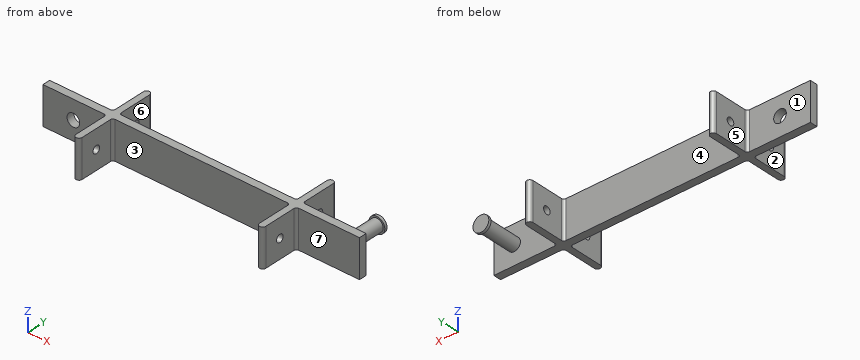
from build123d import *

# Parameters (mm, degrees)
BOSS_EXTRUDE1_DEPTH  = 30
FILLET1_R            = 2
FILLET2_RADIUS       = 2.5
FILLET2_LENGTH       = 30
FILLET3_RADIUS       = 2.5
FILLET3_LENGTH       = 30
FILLET4_R            = 2
SKETCH2_R            = 3
CUT_EXTRUDE4_DEPTH   = 163
SKETCH9_W            = 10
SKETCH9_H            = 6
BOSS_EXTRUDE8_DEPTH  = 30
SKETCH14_W           = 20
SKETCH14_H           = 6
BOSS_EXTRUDE12_DEPTH = 30
FILLET10_RADIUS      = 2.5
FILLET10_LENGTH      = 30
FILLET11_RADIUS      = 2.5
FILLET11_LENGTH      = 30
FILLET12_R           = 2
SKETCH16_R           = 3
CUT_EXTRUDE6_DEPTH   = 200
SKETCH17_W           = 30
SKETCH17_H           = 6
BOSS_EXTRUDE15_DEPTH = 30
SKETCH20_R           = 5
BOSS_EXTRUDE16_DEPTH = 36
SKETCH21_R           = 6.25
BOSS_EXTRUDE17_DEPTH = 2
SKETCH22_R           = 5
CUT_EXTRUDE7_DEPTH   = 10


with BuildPart() as part:
    # Sketch1 → Boss-Extrude1 (new body)
    with BuildSketch(Plane.XY):
        Polygon((-28.863636364, 0), (-48.863636364, 0), (-48.863636364, -30), (-53.863636364, -30), (-53.863636364, 0), (-193.863636364, 0), (-193.863636364, -30), (-198.863636364, -30), (-198.863636364, 0), (-218.863636364, 0), (-218.863636364, 6), (-198.863636364, 6), (-198.863636364, 36), (-193.863636364, 36), (-193.863636364, 6), (-53.863636364, 6), (-53.863636364, 36), (-48.863636364, 36), (-48.863636364, 6), (-28.863636364, 6), align=None)
    extrude(amount=BOSS_EXTRUDE1_DEPTH)

    # Fillet1
    fillet1_edges = [part.edges().sort_by_distance(p)[0] for p in [
        (-198.863636364, 6, 15),
        (-193.863636364, 6, 15),
    ]]
    fillet(fillet1_edges, radius=FILLET1_R)

    # Fillet2: full round fillet: the end face becomes a half cylinder, R = half its width
    fillet2_face = Plane((-196.363636364, 36, 15), x_dir=(0, 0, 1), z_dir=(0, 1, 0))  # on the end face: x along it, z out of the body
    fillet2_slab = fillet2_face.offset(-FILLET2_RADIUS / 2) * Box(FILLET2_LENGTH, 2 * FILLET2_RADIUS, FILLET2_RADIUS, mode=Mode.PRIVATE)  # the body's end, R deep
    fillet2_round = Plane((-196.363636364, 33.5, 15), x_dir=(0, 1, 0), z_dir=(0, 0, 1)) * Cylinder(FILLET2_RADIUS, FILLET2_LENGTH, mode=Mode.PRIVATE)  # its axis R under the face
    add(fillet2_slab - fillet2_round, mode=Mode.SUBTRACT)

    # Fillet3: full round fillet: the end face becomes a half cylinder, R = half its width
    fillet3_face = Plane((-51.363636364, 36, 15), x_dir=(0, 0, 1), z_dir=(0, 1, 0))  # on the end face: x along it, z out of the body
    fillet3_slab = fillet3_face.offset(-FILLET3_RADIUS / 2) * Box(FILLET3_LENGTH, 2 * FILLET3_RADIUS, FILLET3_RADIUS, mode=Mode.PRIVATE)  # the body's end, R deep
    fillet3_round = Plane((-51.363636364, 33.5, 15), x_dir=(0, 1, 0), z_dir=(0, 0, 1)) * Cylinder(FILLET3_RADIUS, FILLET3_LENGTH, mode=Mode.PRIVATE)  # its axis R under the face
    add(fillet3_slab - fillet3_round, mode=Mode.SUBTRACT)

    # Fillet4
    fillet4_edges = [part.edges().sort_by_distance(p)[0] for p in [
        (-53.863636364, 6, 15),
        (-48.863636364, 6, 15),
    ]]
    fillet(fillet4_edges, radius=FILLET4_R)

    # Sketch2 → Cut-Extrude4 (cut)
    with BuildSketch(Plane.ZY.offset(198.863636364)):
        with Locations((15, 21)):
            Circle(SKETCH2_R)
    extrude(amount=-CUT_EXTRUDE4_DEPTH, mode=Mode.SUBTRACT)

    # Sketch9 → Boss-Extrude8 (add)
    with BuildSketch(Plane(origin=(0, 0, 0), x_dir=(-1, 0, 0), z_dir=(0, 0, -1))):
        with Locations((223.863636364, 3)):
            Rectangle(SKETCH9_W, SKETCH9_H)
    extrude(amount=-BOSS_EXTRUDE8_DEPTH)

    # Sketch14 → Boss-Extrude12 (add)
    with BuildSketch(Plane(origin=(0, 0, 0), x_dir=(-1, 0, 0), z_dir=(0, 0, -1))):
        with Locations((238.863636364, 3)):
            Rectangle(SKETCH14_W, SKETCH14_H)
    extrude(amount=-BOSS_EXTRUDE12_DEPTH)

    # Fillet10: full round fillet: the end face becomes a half cylinder, R = half its width
    fillet10_face = Plane((-51.363636364, -30, 15), x_dir=(0, 0, 1), z_dir=(0, -1, 0))  # on the end face: x along it, z out of the body
    fillet10_slab = fillet10_face.offset(-FILLET10_RADIUS / 2) * Box(FILLET10_LENGTH, 2 * FILLET10_RADIUS, FILLET10_RADIUS, mode=Mode.PRIVATE)  # the body's end, R deep
    fillet10_round = Plane((-51.363636364, -27.5, 15), x_dir=(0, -1, 0), z_dir=(0, 0, 1)) * Cylinder(FILLET10_RADIUS, FILLET10_LENGTH, mode=Mode.PRIVATE)  # its axis R under the face
    add(fillet10_slab - fillet10_round, mode=Mode.SUBTRACT)

    # Fillet11: full round fillet: the end face becomes a half cylinder, R = half its width
    fillet11_face = Plane((-196.363636364, -30, 15), x_dir=(0, 0, 1), z_dir=(0, -1, 0))  # on the end face: x along it, z out of the body
    fillet11_slab = fillet11_face.offset(-FILLET11_RADIUS / 2) * Box(FILLET11_LENGTH, 2 * FILLET11_RADIUS, FILLET11_RADIUS, mode=Mode.PRIVATE)  # the body's end, R deep
    fillet11_round = Plane((-196.363636364, -27.5, 15), x_dir=(0, -1, 0), z_dir=(0, 0, 1)) * Cylinder(FILLET11_RADIUS, FILLET11_LENGTH, mode=Mode.PRIVATE)  # its axis R under the face
    add(fillet11_slab - fillet11_round, mode=Mode.SUBTRACT)

    # Fillet12
    fillet12_edges = [part.edges().sort_by_distance(p)[0] for p in [
        (-48.863636364, 0, 15),
        (-53.863636364, 0, 15),
        (-193.863636364, 0, 15),
        (-198.863636364, 0, 15),
    ]]
    fillet(fillet12_edges, radius=FILLET12_R)

    # Sketch16 → Cut-Extrude6 (cut)
    with BuildSketch(Plane(origin=(-48.863636364, 0, 0), x_dir=(0, 0, -1), z_dir=(1, 0, 0))):
        with Locations(Location((-15, -14.75, 0), (0, 0, 90))):
            Circle(SKETCH16_R)
    extrude(amount=-CUT_EXTRUDE6_DEPTH, mode=Mode.SUBTRACT)

    # Sketch17 → Boss-Extrude15 (add)
    with BuildSketch(Plane(origin=(0, 0, 0), x_dir=(-1, 0, 0), z_dir=(0, 0, -1))):
        with Locations((13.863636364, 3)):
            Rectangle(SKETCH17_W, SKETCH17_H)
    extrude(amount=-BOSS_EXTRUDE15_DEPTH)

    # Sketch20 → Boss-Extrude16 (add)
    with BuildSketch(Plane(origin=(0, 0, 0), x_dir=(-1, 0, 0), z_dir=(0, -1, 0))):
        with Locations(Location((14.863636364, -15, 0), (0, 0, 90))):
            Circle(SKETCH20_R)
    extrude(amount=-BOSS_EXTRUDE16_DEPTH)

    # Sketch21 → Boss-Extrude17 (add)
    with BuildSketch(Plane(origin=(0, 36, 0), x_dir=(-1, 0, 0), z_dir=(0, 1, 0))):
        with Locations(Location((14.863636364, 15, 0), (0, 0, 90))):
            Circle(SKETCH21_R)
    extrude(amount=-BOSS_EXTRUDE17_DEPTH)

    # Sketch22 → Cut-Extrude7 (cut)
    with BuildSketch(Plane(origin=(0, 6, 0), x_dir=(1, 0, 0), z_dir=(0, 1, 0))):
        with Locations(Location((-224.863636364, -15, 0), (0, 0, 180))):
            Circle(SKETCH22_R)
    extrude(amount=-CUT_EXTRUDE7_DEPTH, mode=Mode.SUBTRACT)


solid = part.part
Here's how the part is built. I have some questions about the finished solid (model axes, mm). Face numbers are marked on the shaded views. A direction names the side the tool comes from. Round coordinates to 2 decimals unless told otherwise and drop trailing zeros. Order: outer loops, then holes, each group sorted by start corner. A loop starts at its lowest first (then second) coordinate and runs counter-clockwise, first axis right, second up. Notation, with made-up numbers: M 0.25,77.25 L 45.25,77.25 A22 ccw 45.25,103.25 Z; hole C 80,42 d7. An arc over 180 degrees is marked long. One line per question, with ' | ' between items.
1) Imagine slicing it at B-B, the plane z = 15. Count the separate pieces of the cut face and the enclosed holes in it, plus the area to 3 significant figures.
Checked values:
separate pieces: 6 | enclosed holes: 0 | area: 2,220 mm²
2) I need wall thicknesses on line 1 (X direction, y = 12.5, z = 8); line 2 (Y direction, x = -181, z = 1.5); line 3 (X direction, y = 7.5, z = 21). Which ranges of each line are inside material? Lowest first, please.
Checked values:
line 1: x = -198.86 to -193.86, -53.86 to -48.86 | line 2: y = 0 to 6 | line 3: x = -198.93 to -193.8, -53.93 to -48.8
3) We'd pull the mould along X, two halves only. Please class the marked faces 5, 6 and 7: released by +X, released by -X, zero draft, split by the parting line, or undercut.
Checked values:
face 5: released by -X | face 6: undercut | face 7: zero draft
4) Imagine slicing it at D-D, the plane x = -37. Write out the boundary of the cut face in (y, z).
Checked values:
outline: M 0,0 L 6,0 L 6,30 L 0,30 Z
5) On a 3-axis mill with a long thin cutter (end or side, diameter ignored), from which of +Z, -Z, +X, -X, +Y, -Y can I reach the whole of each face in a straight line? I mean the marked faces 1, 2, 3 and 4. Say none if no direction works.
Checked values:
face 1: +Z, -Z, -X, +Y | face 2: +Z, -Z, -X, -Y | face 3: +Z, -Z, -Y | face 4: +Z, -Z, +Y
6) I'm going to push flat-ended pins straight in: pin 1 Ø13 at (y, z) = (24, 9.5) entering from -X; pin 2 Ø12 at (y, z) = (-15.5, 12) entering from +X; pin 3 Ø8 at (y, z) = (21, 15) entering from +X. Where does each tip first touch, or does it pass through?
Checked values:
pin 1: stops at x = -198.86 | pin 2: stops at x = -48.86 | pin 3: stops at x = -9.86
7) Imagine slicing it at C-C, the plane y = 21. Write out the boundary of the cut face in (x, z), plus the area to 3 significant figures.
Checked values:
outline: M -198.86,0 L -193.86,0 L -193.86,12 L -198.86,12 Z; M -198.86,18 L -193.86,18 L -193.86,30 L -198.86,30 Z; M -53.86,0 L -48.86,0 L -48.86,12 L -53.86,12 Z; M -53.86,18 L -48.86,18 L -48.86,30 L -53.86,30 Z; C -14.86,15 d10 | area: 319 mm²
8) Imagine slicing it at A-A, the plane y = -23. Write out the boundary of the cut face in (x, z).
Checked values:
outline: M -198.86,0 L -193.86,0 L -193.86,30 L -198.86,30 Z; M -53.86,0 L -48.86,0 L -48.86,30 L -53.86,30 Z
